Design review of the part built by this model. Coordinates are the model's own, in mm. Face numbers are marked on the shaded views. A direction names the side the tool comes from. Round coordinates to 2 decimals unless told otherwise and drop trailing zeros. Loops run counter-clockwise (first coordinate to the right, second up) from the corner with the lowest first, then second, coordinate; pieces in that order, holes last. Notation, with made-up numbers: (33.5, -3.75) - (43.5, -3.75) arc R15 ccw to (43.5, 10.25) - close; hole circle Ø1 at (34.5, 54.5). An arc over 180 degrees is marked (long way). Use one line per item in the form item = value. Start each with the question number.
(1) We need section B-B, the plane x = 0. Write out the cut boundary in (y, z).
(2) We need section D-D, the plane y = 23. Write out the cut boundary in (x, z), then the cut area to 3 significant figures.
(3) Machinability: for the marked faces 1, 2 and 3, which of the approach directions +Z, -Z, +X, -X, +Y, -Y give a long, thin tool a straight path to every point of the face, cutting with its end or side? Answer none if there is none.
(4) The part is to be moulded in two halves that separate along Z. For the marked faces 4, 5 and 6, say which applies: released by +Z, released by -Z, zero draft, split by the parting line, or undercut.
(5) We need section A-A, the plane z = 1. Write out the cut boundary in (x, y).
(6) Wall thickness on probe 1 along Y at (x, z) = (-0.25, -1.5); probe 2 along Y at (x, z) = (-1, 1); probe 3 along Y at (x, z) = (1.75, 1.75): over which ranges is each line inside the solid? List them lowest first. Write a range as [from, to].
(7) We need section C-C, the plane z = -1. Write out the cut boundary in (x, y), then the cut area to 3 significant figures.
(8) For pin 1 (1.1 mm diameter, centred on x = 0.5, y = 24.5, fed in from +Z); pin 2 (1 mm diameter, centred on x = 2, y = 24.5, fed in from -Z); pin 3 (0.6 mm diameter, centred on x = -2, y = 25.5, fed in from +Z); pin 4 (3.5 mm diameter, centred on y = 25.5, z = 1, fed in from -X), all flat-tipped, find the tip position at first contact; note any pin that passes through.
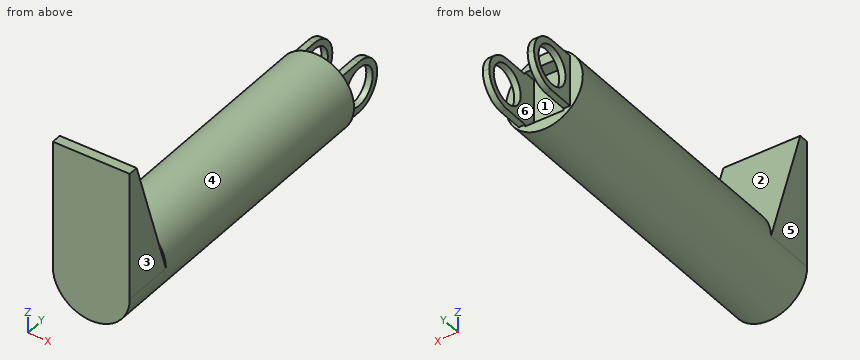
from build123d import *

# Parameters (mm, degrees)
SKETCH1_R           = 3
BOSS_EXTRUDE1_DEPTH = 25
SKETCH2_W           = 4
SKETCH2_H           = 4
SKETCH2_W_2         = 3
SKETCH2_H_2         = 3
BOSS_EXTRUDE2_DEPTH = 4
SKETCH3_W           = 3
SKETCH3_H           = 4.288213466
CUT_EXTRUDE1_DEPTH  = 5
SKETCH4_R           = 1.5
CUT_EXTRUDE2_DEPTH  = 5
FILLET1_R           = 2
SKETCH5_W           = 6
SKETCH5_H           = 4.032898641
BOSS_EXTRUDE3_DEPTH = 10
CUT_EXTRUDE4_DEPTH  = 10


with BuildPart() as part:
    # Sketch1 → Boss-Extrude1 (new body)
    with BuildSketch(Plane(origin=(0, 0, 0), x_dir=(1, 0, 0), z_dir=(0, 1, 0))):
        with Locations(Location((0, 0, 0), (0, 0, 270))):
            Circle(SKETCH1_R)
    extrude(amount=BOSS_EXTRUDE1_DEPTH)

    # Sketch2 → Boss-Extrude2 (add)
    with BuildSketch(Plane(origin=(0, 25, 0), x_dir=(1, 0, 0), z_dir=(0, 1, 0))):
        Rectangle(SKETCH2_W, SKETCH2_H)
        Rectangle(SKETCH2_W_2, SKETCH2_H_2, mode=Mode.SUBTRACT)
    extrude(amount=BOSS_EXTRUDE2_DEPTH)

    # Sketch3 → Cut-Extrude1 (cut)
    with BuildSketch(Plane(origin=(0, 29, 0), x_dir=(1, 0, 0), z_dir=(0, 1, 0))):
        Rectangle(SKETCH3_W, SKETCH3_H)
    extrude(amount=-CUT_EXTRUDE1_DEPTH, mode=Mode.SUBTRACT)

    # Sketch4 → Cut-Extrude2 (cut)
    with BuildSketch(Plane.ZY.offset(2)):
        with Locations((0, 27)):
            Circle(SKETCH4_R)
    extrude(amount=-CUT_EXTRUDE2_DEPTH, mode=Mode.SUBTRACT)

    # Fillet1
    fillet1_edges = [part.edges().sort_by_distance(p)[0] for p in [
        (1.75, 29, 2),
        (1.75, 29, -2),
        (-1.75, 29, -2),
        (-1.75, 29, 2),
    ]]
    fillet(fillet1_edges, radius=FILLET1_R - 0.0001)  # a hair under: the kernel refuses the full size

    # Sketch5 → Boss-Extrude3 (add)
    with BuildSketch(Plane.XY):
        with Locations((0, 2.016449321)):
            Rectangle(SKETCH5_W, SKETCH5_H)
    extrude(amount=BOSS_EXTRUDE3_DEPTH)

    # Sketch6 → Cut-Extrude4 (cut)
    with BuildSketch(Plane.ZY.offset(3)):
        Polygon((0, 4.032898641), (10, 0.769169486), (10, 4.032898641), align=None)
    extrude(amount=-CUT_EXTRUDE4_DEPTH, mode=Mode.SUBTRACT)


solid = part.part
Data:
q1.outline = (0, -3) - (25, -3) - (25, -2.14) - (24, -2.14) - (24, 2.14) - (25, 2.14) - (25, 3) - (4.03, 3) - (4.03, 0) - (0.77, 10) - (0, 10) - close
q2.outline = circle Ø6 at (0, 0)
q2.area = 28.3 mm^2
q3.face_1 = +Y
q3.face_2 = +Z, +X, -X
q3.face_3 = +Z, -Z, +X, +Y, -Y
q4.face_4 = split by the parting line
q4.face_5 = zero draft
q4.face_6 = undercut
q5.outline = (-3, 0) - (3, 0) - (3, 3.71) - (-3, 3.71) - close; (-2.83, 4.03) - (2.83, 4.03) - (2.83, 25) - (2, 25) - (2, 25.88) - (1.5, 25.88) - (1.5, 24) - (-1.5, 24) - (-1.5, 25.88) - (-2, 25.88) - (-2, 25) - (-2.83, 25) - close; (-2, 28.12) - (-1.5, 28.12) - (-1.5, 28.73) - (-2, 28.73) - close; (1.5, 28.12) - (2, 28.12) - (2, 28.73) - (1.5, 28.73) - close
q6.probe_1 = [0, 24]
q6.probe_2 = [0, 3.71], [4.03, 24]
q6.probe_3 = [0, 3.46], [4.03, 27.97]
q7.outline = (-2.83, 0) - (2.83, 0) - (2.83, 25) - (2, 25) - (2, 25.88) - (1.5, 25.88) - (1.5, 24) - (-1.5, 24) - (-1.5, 25.88) - (-2, 25.88) - (-2, 25) - (-2.83, 25) - close; (-2, 28.12) - (-1.5, 28.12) - (-1.5, 28.73) - (-2, 28.73) - close; (1.5, 28.12) - (2, 28.12) - (2, 28.73) - (1.5, 28.73) - close
q7.area = 140 mm^2
q8.pin_1 = 3
q8.pin_2 = -2.6
q8.pin_3 = 2
q8.pin_4 = -3
